from build123d import *

# Parameters (mm, degrees)
SKETCH1_R           = 40
BOSS_EXTRUDE1_DEPTH = 350
SKETCH2_R           = 15
BOSS_EXTRUDE2_DEPTH = 50
BOSS_EXTRUDE4_START = 70
SKETCH4_R           = 15
BOSS_EXTRUDE4_DEPTH = 70
CUT_EXTRUDE1_DEPTH  = 20
FILLET2_R           = 0.1


with BuildPart() as part:
    # Sketch1 → Boss-Extrude1 (new body)
    with BuildSketch(Plane.XY):
        Circle(SKETCH1_R)
    extrude(amount=BOSS_EXTRUDE1_DEPTH)

    # Sketch2 → Boss-Extrude2 (add)
    with BuildSketch(Plane.XY.offset(350)):
        Circle(SKETCH2_R)
    extrude(amount=BOSS_EXTRUDE2_DEPTH)

    # Sketch4 → Boss-Extrude4 (add)
    with BuildSketch(Plane(origin=(0, 0, 0), x_dir=(-1, 0, 0), z_dir=(0, 0, -1)).offset(BOSS_EXTRUDE4_START)):
        with Locations(Location((0, 0, 0), (0, 0, 180))):
            Circle(SKETCH4_R)
    extrude(amount=-BOSS_EXTRUDE4_DEPTH)

    # Sketch5 → Cut-Extrude1 (cut)
    with BuildSketch(Plane(origin=(0, 0, -70), x_dir=(-1, 0, 0), z_dir=(0, 0, -1))):
        with BuildLine():
            Line((-2, 11.324751653), (-2, 14.866068747))
            ThreePointArc((-2, 14.866068747), (0, 15), (2, 14.866068747))
            Line((2, 14.866068747), (2, 11.324751653))
            ThreePointArc((2, 11.324751653), (0, 11.5), (-2, 11.324751653))
        make_face()
    extrude(amount=-CUT_EXTRUDE1_DEPTH, mode=Mode.SUBTRACT)

    # Fillet2
    fillet2_edges = [part.edges().sort_by_distance(p)[0] for p in [
        (-9.874208829, -11.291589791, -70),
    ]]
    fillet(fillet2_edges, radius=FILLET2_R)


solid = part.part
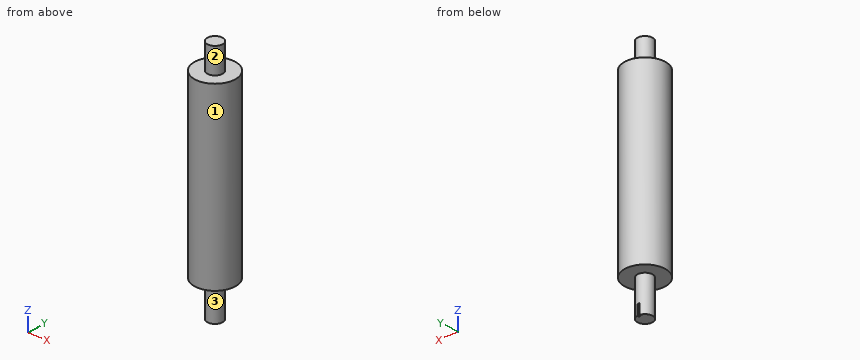
Can you work these out from the model? Positions are in its coordinate system, mm. Face numbers are marked on the shaded views. A direction names the side the tool comes from. Give positions to 0.01 mm unless a question says otherwise; leave off trailing zeros. Order: outer loops, then holes, each group sorted by start corner. A loop starts at its lowest first (then second) coordinate and runs counter-clockwise, first axis right, second up. Notation, with made-up numbers: M 23.5,-10 L 59.5,-10 A24 ccw 59.5,1 Z; hole C 80,85 d9. An arc over 180 degrees is marked long. One line per question, with ' | ' between items.
Item 1: Suppose I cut it at D-D, the plane z = 370.5. Write out the boundary of the cut face in (x, y).
Answer block:
outline: C 0,0 d30
Item 2: Suppose I cut it at A-A, the plane y = 0. Write out the boundary of the cut face in (x, z), then the cut area to 3 significant figures.
Answer block:
outline: M -40,0 L -15,0 L -15,-69.9 A0.1 ccw -14.9,-70 L 14.9,-70 A0.1 ccw 15,-69.9 L 15,0 L 40,0 L 40,350 L 15,350 L 15,400 L -15,400 L -15,350 L -40,350 Z | area: 31,600 mm2
Item 3: Suppose I cut it at B-B, the plane z = 41. Write out the boundary of the cut face in (x, y), then the cut area to 3 significant figures.
Answer block:
outline: C 0,0 d80 | area: 5,030 mm2
Item 4: For the marked faces 1, 2 and 3, which set-ups out of +Z, -Z, +X, -X, +Y, -Y let a thin tool reach every point of the face, with its end or its side?
Answer block:
face 1: +Z, -Z | face 2: +Z | face 3: -Z
Item 5: Please list where these lines run through material, in increasing order: L1, parallel to Z at x = 17, y = -17.5; L2, parallel to X at y = -2, z = 192; L3, parallel to Y at x = 0, z = -44.
Answer block:
L1: z = 0 to 350 | L2: x = -39.95 to 39.95 | L3: y = -15 to 15
Item 6: I'm going to push flat-ended pins straight in: pin 1 Ø3 at (y, z) = (13.5, -55.5) entering from +X; pin 2 Ø6 at (x, z) = (16, 180.5) entering from -Y; pin 3 Ø4 at (y, z) = (13.5, 299.5) entering from -X. Where does each tip first touch, or does it pass through?
Answer block:
pin 1: stops at x = 9 | pin 2: stops at y = -37.83 | pin 3: stops at x = -38.31
Item 7: Suppose I cut it at C-C, the plane x = -28. Write out the boundary of the cut face in (y, z).
Answer block:
outline: M -28.57,0 L 28.57,0 L 28.57,350 L -28.57,350 Z
